Answer from the drawing. Dimensions are ordinates in mm from the lowest x, y and z of the part. Give positions to 0.01 mm unless a question says otherwise; leave off trailing zeros. Loops run counter-clockwise (first coordinate to the right, second up) from the corner with the lowest first, then second, coordinate; pieces in that order, holes last. Notation, with made-up numbers: (-16, -4) - (28, -4) arc R30 ccw to (28, 25) - close; hole circle Ø10 at (65, -12). An arc over 180 degrees is marked (long way). Answer as CSV lines item,"result". Start each with the question number.
1) A cutting plane is placed at A-A (y = 2.2). Determine the outline of the cut face in (x, z).
2) Find the intervals of material crossed by line 1 along X through (y, z) = (1.6, 50.5); line 2 along Z through (x, y) = (37.5, 1.5), in increasing order.
3) Flat-ended cylindrical pins translate along their axes: pin 1 (1 mm diameter, centred on y = 2, z = 27, fed in from -X); pin 2 (1 mm diameter, centred on x = 25, y = 2, fed in from +Z). Find the tip coordinate at first contact, or state that the pin passes through.
4) A cutting plane is placed at B-B (x = 41). Determine the outline of the cut face in (y, z).
5) A cutting plane is placed at C-C (z = 19.5). Determine the outline of the cut face in (x, y).
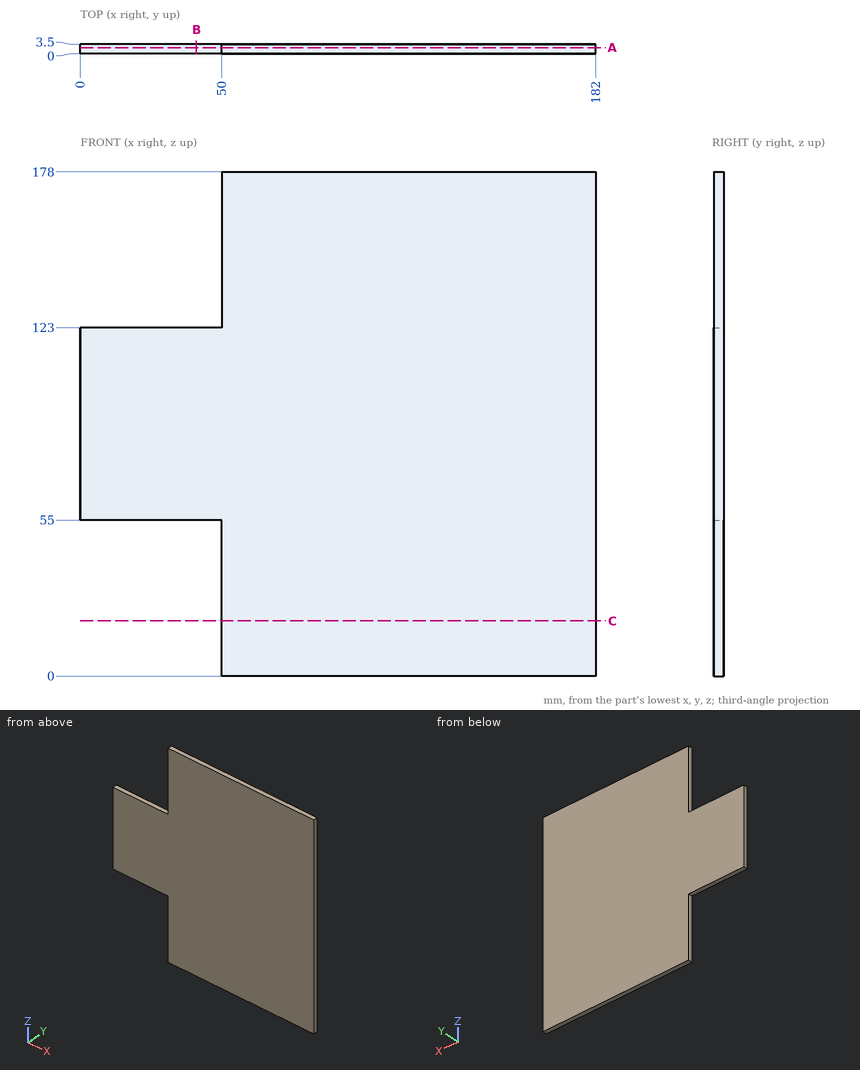
Ans:
1,outline,"(0, 55) - (50, 55) - (50, 0) - (182, 0) - (182, 178) - (50, 178) - (50, 123) - (0, 123) - close"
2,line 1,"50 to 182"
2,line 2,"55 to 123"
3,pin 1,"x = 50"
3,pin 2,"z = 123"
4,outline,"(0, 55) - (3.5, 55) - (3.5, 123) - (0, 123) - close"
5,outline,"(50, 0) - (182, 0) - (182, 3.5) - (50, 3.5) - close"
